Here's how the part is built. I have some questions about the finished solid (model axes, mm). A direction names the side the tool comes from. Coordinates: 2 decimals unless noted, no trailing zeros. Loops run counter-clockwise (first coordinate to the right, second up) from the corner with the lowest first, then second, coordinate; pieces in that order, holes last. Notation, with made-up numbers: M 72.5,-20.75 L 130.5,-20.75 A19 cw 130.5,-5.75 Z; hole C 40.5,9 d11. An arc over 180 degrees is marked long. Use one line per item in the form item = value. Start each with the question number.
(1) Please list where these lines run through material, in increasing order: L1, parallel to Y at x = -103, z = -5.75; L2, parallel to Z at x = -22, y = 28.5; L3, parallel to X at y = 2, z = -13.
(2) Imagine slicing it at C-C, the plane z = -13.75. Please give me the cut outline in (x, y).
(3) Imagine slicing it at B-B, the plane x = -25. Please give me the cut outline in (y, z), and give its area (3 significant figures).
(4) Will these pins go through, and if not, where does the flat tip stop? P1, Ø1.5, axis at x = -43, y = 24, coming from the -Z side; P2, Ø2, axis at x = -34.5, z = -17.5, coming from the +Y side; P3, Ø5, axis at x = -74.5, z = -11, coming from the -Y side; P4, Ø1, axis at x = -126.5, z = -19.5, coming from the +Y side.
(5) On a 3-axis mill with a long thin cutter (end or side, diameter ignored), from which of +Z, -Z, +X, -X, +Y, -Y can I reach the whole of each face in a straight line? I mean faces 1 (the flat face through (-91, 17, -1)), 2 (the flat face through (-89, 1, -10)), 3 (the flat face through (11.44, 17.08, -10.72)). Say none if no direction works.
(6) Imagine slicing it at A-A, the plane y = 12.5. Please give me the cut outline in (x, z), and give its area (3 significant figures).
```python
from build123d import *

# Parameters (mm, degrees)
SKETCH2_W                    = 180
SKETCH2_H                    = 32
BASE_FLANGE1_DEPTH           = 1
EDGE_FLANGE1_STRIP_W         = 5.4732
EDGE_FLANGE1_STRIP_H         = 1
EDGE_FLANGE1_STRIP_CUT_DEPTH = 180
EDGE_FLANGE1_DEPTH           = 180
EDGE_FLANGE2_DEPTH           = 30.2634
FILLET1_R                    = 2


# Sheet-metal steps are written as plain solids
with BuildPart() as part:
    # Sketch2 → Base-Flange1 (new body)
    with BuildSketch(Plane.XY):
        with Locations((-90, 16)):
            Rectangle(SKETCH2_W, SKETCH2_H)
    extrude(amount=-BASE_FLANGE1_DEPTH)

    # Edge-Flange1 strip (across the edge) → Edge-Flange1 strip cut (cut)
    with BuildSketch(Plane(origin=(0, 0, -1), x_dir=(0, 1, 0), z_dir=(-1, 0, 0))):
        with Locations((-1, -0.5)):
            Rectangle(EDGE_FLANGE1_STRIP_W, EDGE_FLANGE1_STRIP_H)
    extrude(amount=EDGE_FLANGE1_STRIP_CUT_DEPTH, mode=Mode.SUBTRACT)

    # Edge-Flange1 section (across the edge) → Edge-Flange1 (add)
    with BuildSketch(Plane(origin=(0, 0, -1), x_dir=(0, 1, 0), z_dir=(-1, 0, 0))):
        with BuildLine():
            Line((0, 0.7366), (0, 17))
            Line((0, 17), (1, 17))
            Line((1, 17), (1, 0.7366))
            ThreePointArc((1, 0.7366), (1.215745145, 0.215745145), (1.7366, 0))
            Line((1.7366, 0), (1.7366, -1))
            ThreePointArc((1.7366, -1), (0.508638364, -0.491361636), (0, 0.7366))
        make_face()
    extrude(amount=EDGE_FLANGE1_DEPTH)

    # Edge-Flange2 section (across the edge) → Edge-Flange2 (add)
    with BuildSketch(Plane(origin=(0.30510971, 32, -1), x_dir=(-0.7071067811865438, 0, -0.7071067811865512), z_dir=(0, -1, 0))):
        with BuildLine():
            Line((-1, 0.30510971), (-1, 29.585786438))
            Line((-1, 29.585786438), (0, 29.585786438))
            Line((0, 29.585786438), (0, 0.30510971))
            ThreePointArc((0, 0.30510971), (0.056070336, 0.023225094), (0.215745145, -0.215745145))
            Line((0.215745145, -0.215745145), (-0.491361636, -0.922851926))
            ThreePointArc((-0.491361636, -0.922851926), (-0.867809196, -0.359458339), (-1, 0.30510971))
        make_face()
    extrude(amount=EDGE_FLANGE2_DEPTH)

    # Fillet1
    fillet1_edges = [part.edges().sort_by_distance(p)[0] for p in [
        (0, 0.5, -18),
        (-180, 0.5, -18),
        (21.578973317, 32, -21.566756826),
        (21.578973317, 1.7366, -21.566756826),
        (-180, 32, -0.5),
    ]]
    fillet(fillet1_edges, radius=FILLET1_R)


solid = part.part
```
Answer:
q1.L1 = 0 to 1
q1.L2 = -1 to 0
q1.L3 = 12.31 to 13.72
q2.outline = M -180,0 L 0,0 L 0,1 L -180,1 Z; M 13.06,1.74 L 14.47,1.74 L 14.47,32 L 13.06,32 Z
q3.outline = M 0,-18 L 1,-18 L 1,-1.74 A0.74 cw 1.74,-1 L 32,-1 L 32,0 L 1.74,0 A1.74 ccw 0,-1.74 Z
q3.area = 48.5 mm²
q4.P1 = -1
q4.P2 = 1
q4.P3 = 0
q4.P4 = through
q5.face_1 = -Z, -X, +Y
q5.face_2 = -Z, +X, -X, +Y
q5.face_3 = +Z, +X, +Y, -Y
q6.outline = M -180,-1 L 0,-1 A0.74 cw 0.52,-1.22 L 21.23,-21.92 L 21.93,-21.21 L 1.23,-0.51 A1.74 ccw 0,0 L -180,0 Z
q6.area = 210 mm²
